Design review of the part built by this model. Coordinates are the model's own, in mm. A direction names the side the tool comes from. Give positions to 0.01 mm unless a question says otherwise; leave off trailing zeros. Order: outer loops, then holes, each group sorted by start corner. A loop starts at its lowest first (then second) coordinate and runs counter-clockwise, first axis right, second up. Notation, with made-up numbers: (9.5, 76.25) -> (29.5, 76.25) arc R18 cw to (29.5, 106.25) -> close; hole circle Ø2 at (43, 4.5). An arc over 180 degrees is marked (long way). Use a Markdown table: item, result. Add a question column.
```python
from build123d import *

# Parameters (mm, degrees)
F0_W     = 6
F0_H     = 12
F0_R     = 2
F1_DEPTH = 6


with BuildPart() as f1:
    # F0 (on Front) → F1 (new body)
    with BuildSketch(Plane.XZ):
        with BuildLine():
            Line((1, 39), (0, 39))
            Line((0, 39), (-1, 39))
            ThreePointArc((-1, 39), (-4.535534, 37.535534), (-6, 34))
            Line((-6, 34), (-6, 32))
            ThreePointArc((-6, 32), (-10.393398, 21.393398), (-21, 17))
            Line((-21, 17), (-44.63, 17))
            ThreePointArc((-44.63, 17), (-55.236602, 21.393398), (-59.63, 32))
            Line((-59.63, 32), (-59.63, 34))
            ThreePointArc((-59.63, 34), (-61.094466, 37.535534), (-64.63, 39))
            Line((-64.63, 39), (-66.63, 39))
            ThreePointArc((-66.63, 39), (-70.165534, 37.535534), (-71.63, 34))
            Line((-71.63, 34), (-71.63, 0))
            Line((-71.63, 0), (-59.63, 0))
            ThreePointArc((-59.63, 0), (-58.165534, 3.535534), (-54.63, 5))
            Line((-54.63, 5), (0, 5))
            Line((0, 5), (54.63, 5))
            ThreePointArc((54.63, 5), (58.165534, 3.535534), (59.63, 0))
            Line((59.63, 0), (71.63, 0))
            Line((71.63, 0), (71.63, 34))
            ThreePointArc((71.63, 34), (70.165534, 37.535534), (66.63, 39))
            Line((66.63, 39), (64.63, 39))
            ThreePointArc((64.63, 39), (61.094466, 37.535534), (59.63, 34))
            Line((59.63, 34), (59.63, 32))
            ThreePointArc((59.63, 32), (55.236602, 21.393398), (44.63, 17))
            Line((44.63, 17), (21, 17))
            ThreePointArc((21, 17), (10.393398, 21.393398), (6, 32))
            Line((6, 32), (6, 34))
            ThreePointArc((6, 34), (4.535534, 37.535534), (1, 39))
        make_face()
        with Locations((-65.63, 14)):
            Rectangle(F0_W, F0_H, mode=Mode.SUBTRACT)
        Polygon((-6, 14), (0, 14), (6, 14), (6, 8), (0, 8), (-6, 8), align=None, mode=Mode.SUBTRACT)
        with Locations((65.63, 14)):
            Rectangle(F0_W, F0_H, mode=Mode.SUBTRACT)
        with Locations((-65.63, 33)):
            Circle(F0_R, mode=Mode.SUBTRACT)
        with BuildLine():
            ThreePointArc((0, 31), (-2, 33), (0, 35))
            ThreePointArc((0, 35), (2, 33), (0, 31))
        make_face(mode=Mode.SUBTRACT)
        with Locations((65.63, 33)):
            Circle(F0_R, mode=Mode.SUBTRACT)
    extrude(amount=F1_DEPTH)


solid = f1.part
```
1) The part is to be moulded in two halves that separate along Z. For faces 1 (the flat face through (33, -3, 17)), 2 (the flat face through (0, -3, 8)), 3 (the flat face through (-71.63, -3, 17)), say which applies: +Z half, -Z half, draft (parallel to the pull), parting line (faces both ways), or undercut.
2) For L1, parallel to X at y = -0.15, z = 15.5; L2, parallel to X at y = -1.65, z = 12.5; L3, parallel to Z at x = -65.63, y = -4.2, list the stretches that pass through material, from the lowest coordinate up. Write a range as [from, to].
3) Machinability: for faces 4 (the flat face through (-1, -3, 5)), 5 (the flat face through (66, -3, 20)), 6 (the cylindrical face through (-70.1, -3, 37.6)), 7 (the cylindrical face through (-55.12, -2.96, 21.28)), which of the approach directions +Z, -Z, +X, -X, +Y, -Y give a long, thin tool a straight path to every point of the face, cutting with its end or side? Answer none if there is none.
4) Add section A-A (y = -4.7). Give the number of separate pieces and of enclosed holes in the cut face, then the cut area to 3 significant figures.
5) Add section B-B (x = 15). Give the boundary of the cut face in (y, z), then the cut area to 3 significant figures.
6) Insertion check: pin 1 (3.5 mm diameter, centred on x = 0, z = 33, fed in from +Y); pin 2 (1 mm diameter, centred on x = -25.5, y = -5, fed in from +Z); pin 3 (1 mm diameter, centred on x = 53, y = -1, fed in from -Z). Each pin has a flat end and moves straight along its axis. Give the tip position at first contact, or say it passes through.
Worked answers:
| question | item | result |
|---|---|---|
| 1 | face 1 | +Z half |
| 1 | face 2 | undercut |
| 1 | face 3 | draft |
| 2 | L1 | [-71.63, -68.63], [-62.63, 62.63], [68.63, 71.63] |
| 2 | L2 | [-71.63, -68.63], [-62.63, -6], [6, 62.63], [68.63, 71.63] |
| 2 | L3 | [0, 8], [20, 31], [35, 39] |
| 3 | face 4 | -Z, +Y, -Y |
| 3 | face 5 | +Y, -Y |
| 3 | face 6 | +Z, -X, +Y, -Y |
| 3 | face 7 | +Z, +Y, -Y |
| 4 | separate pieces | 1 |
| 4 | enclosed holes | 6 |
| 4 | area | 2,550 mm^2 |
| 5 | outline | (-6, 5) -> (0, 5) -> (0, 18.25) -> (-6, 18.25) -> close |
| 5 | area | 79.5 mm^2 |
| 6 | pin 1 | through |
| 6 | pin 2 | z = 17 |
| 6 | pin 3 | z = 5 |
